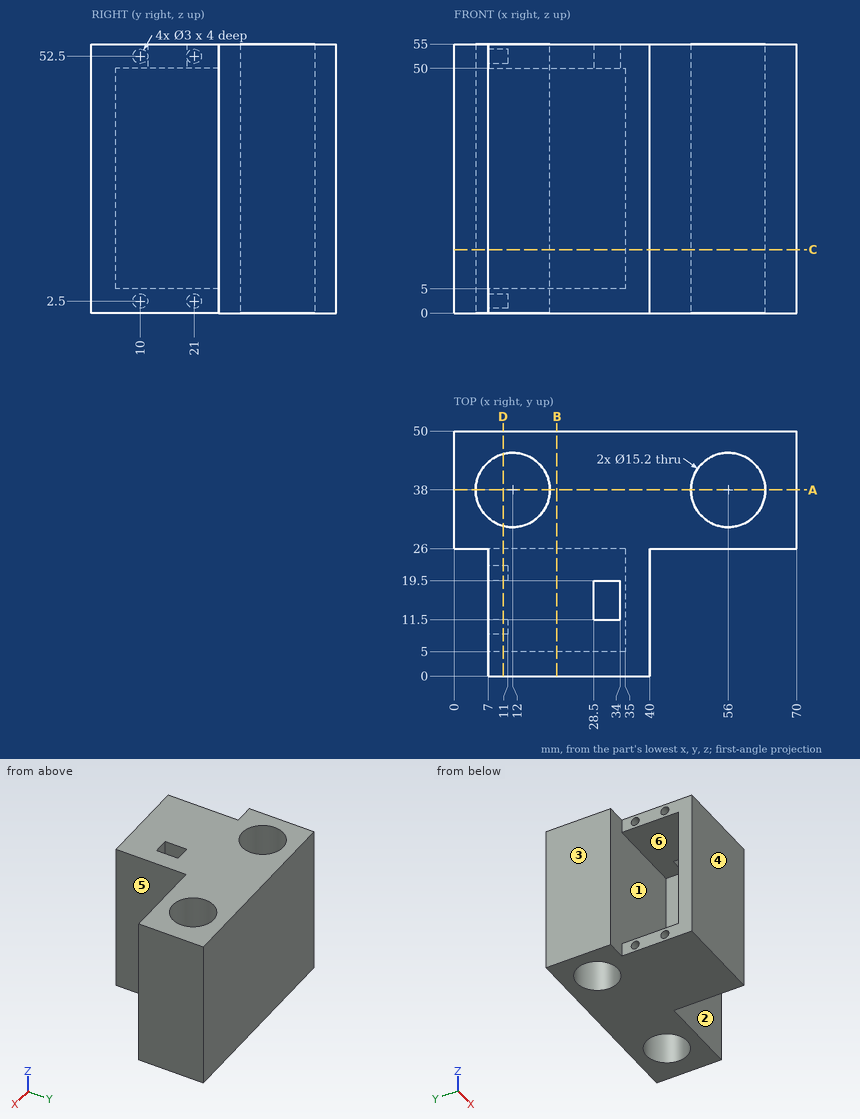
Could you check a few things on this drawing? It's one solid part, dimensions in mm from its lowest x, y, z. A direction names the side the tool comes from. Round coordinates to 2 decimals unless told otherwise and drop trailing zeros. Loops run counter-clockwise (first coordinate to the right, second up) from the corner with the lowest first, then second, coordinate; pieces in that order, holes last. Notation, with made-up numbers: M 88,48.5 L 101,48.5 A27 cw 101,86.5 Z; hole C 80,5 d2. An arc over 180 degrees is marked long. Write each question's results on one line, items separated by ' | '. Start each with the question number.
(1) I want a section at A-A (y = 38). Please give me the cut outline in (x, z).
(2) If I drill on probe 1 along X at (y, z) = (38, 13.5); probe 2 along Y at (x, z) = (12, 41); probe 3 along X at (y, z) = (41, 50), over which ranges is the centre line in solid material (lowest first)? Write a range as from..to.
(3) I want a section at C-C (z = 13). Please give me the cut outline in (x, y), then the cut area to 3 significant figures.
(4) I want a section at D-D (x = 10). Please give me the cut outline in (y, z).
(5) Will these pins go through, and if not, where does the flat tip stop? P1, Ø0.9, axis at y = 20.5, z = 2.5, coming from the -X side; P2, Ø5, axis at y = 21, z = 2.5, coming from the -X side; P3, Ø4, axis at y = 10, z = 2.5, coming from the +X side.
(6) On a 3-axis mill with a long thin cutter (end or side, diameter ignored), from which of +Z, -Z, +X, -X, +Y, -Y can I reach the whole of each face in a straight line? I mean the marked faces 1, 2 and 3. Say none if no direction works.
(7) I want a section at B-B (x = 21). Please give me the cut outline in (y, z).
(8) Thinking about a two-plate mould opening in Y: for the marked faces 4, 5 and 6, which applies, pulls with the +Y half, pulls with the -Y half, needs draft (parallel to the pull), parting line crosses it, or undercut?
Solved:
1) outline: M 0,0 L 4.4,0 L 4.4,55 L 0,55 Z; M 19.6,0 L 48.4,0 L 48.4,55 L 19.6,55 Z; M 63.6,0 L 70,0 L 70,55 L 63.6,55 Z
2) probe 1: x = 0..4.4, 19.6..48.4, 63.6..70 | probe 2: y = 0..5, 26..30.4, 45.6..50 | probe 3: x = 0..5.02, 18.98..49.02, 62.98..70
3) outline: M 0,26 L 35,26 L 35,5 L 7,5 L 7,0 L 40,0 L 40,26 L 70,26 L 70,50 L 0,50 Z; hole C 12,38 d15.2; hole C 56,38 d15.2 | area: 1,590 mm²
4) outline: M 0,0 L 30.67,0 L 30.67,55 L 0,55 Z; M 45.33,0 L 50,0 L 50,55 L 45.33,55 Z; hole M 5,5 L 26,5 L 26,50 L 5,50 Z; hole C 10,2.5 d3; hole C 10,52.5 d3; hole C 21,2.5 d3; hole C 21,52.5 d3
5) P1: stops at x = 11 | P2: stops at x = 7 | P3: stops at x = 40
6) face 1: -X | face 2: +Z, -Z, +X, -Y | face 3: +Z, -Z, -X, +Y, -Y
7) outline: M 0,0 L 50,0 L 50,55 L 0,55 Z; hole M 5,5 L 26,5 L 26,50 L 5,50 Z
8) face 4: pulls with the -Y half | face 5: needs draft | face 6: undercut
